Verification items for the finished model (mm, model axes). Face numbers are marked on the shaded views. A direction names the side the tool comes from. Give positions to 0.01 mm unless a question says otherwise; leave off trailing zeros. Order: outer loops, then holes, each group sorted by start corner. A loop starts at its lowest first (then second) coordinate and runs counter-clockwise, first axis right, second up. Notation, with made-up numbers: (-10.5, 23.5) -> (-1.5, 23.5) arc R5 ccw to (-1.5, 29.5) -> close; hole circle Ø11 at (89, 7.25). An arc over 180 degrees is marked (long way). Write each question's results on one line, items separated by ' | '. Start each with the question number.
1. Depth check by flat-ended pin: pin 1 Ø3 at (x, z) = (9.5, 8) entering from +Y; pin 2 Ø3 at (x, z) = (10.5, 1.5) entering from +Y; pin 3 Ø4 at (y, z) = (9, 2) entering from -X; pin 4 Ø2 at (x, z) = (10, 7) entering from +Y. Enter the tip coordinate at first touch or a pass-through.
2. Mould release check, pull along Y, two halves, no side actions. Record for the marked faces 4, 5, 6 and 7: +Y half, -Y half, draft (parallel to the pull), parting line (faces both ways), or undercut.
3. Cross-section at D-D, the plane y = 13. Enter the section's corners in (x, z).
4. Material ranges on L1, parallel to X at y = -13.05, z = 3; L2, parallel to X at y = -13.85, z = 3; L3, parallel to Z at x = -10, y = -13, recorded low to high. Write a range as from..to.
5. Cross-section at A-A, the plane x = 15. Enter the section's corners in (y, z).
6. Cross-section at C-C, the plane x = -10. Enter the section's corners in (y, z), then the cut area to 3 significant figures.
7. Cross-section at B-B, the plane z = 3. State how many separate pieces and enclosed holes the cut face has, then the cut area to 3 significant figures.
8. Set-up check for the marked faces 1, 2 and 3: record each of +Z, -Z, +X, -X, +Y, -Y from which the full face is reachable in a straight line by a thin tool's end or side.
from build123d import *

# Parameters (mm, degrees)
SKETCH1_R           = 4.5
BOSS_EXTRUDE1_DEPTH = 5
SKETCH2_W           = 5
SKETCH2_H           = 2.5
BOSS_EXTRUDE2_DEPTH = 5
SKETCH3_W           = 7.5
SKETCH3_H           = 2.5
BOSS_EXTRUDE3_DEPTH = 5
SKETCH4_W           = 7.5
SKETCH4_H           = 2.5
BOSS_EXTRUDE4_DEPTH = 5
SKETCH5_R           = 1.65
CUT_EXTRUDE1_DEPTH  = 5
FILLET1_R           = 2
FILLET2_R           = 2
FILLET3_R           = 2
FILLET4_R           = 10
FILLET5_R           = 5
FILLET6_R           = 1


with BuildPart() as part:
    # Sketch1 → Boss-Extrude1 (new body)
    with BuildSketch(Plane.XY):
        with BuildLine():
            Line((-7.5, 15), (-5.646592756, 12.528790341))
            ThreePointArc((-5.646592756, 12.528790341), (0, 16.5), (5.646592756, 12.528790341))
            Line((5.646592756, 12.528790341), (7.5, 15))
            Line((7.5, 15), (12.5, 15))
            Line((12.5, 15), (12.5, 10))
            Line((12.5, 10), (5, 0))
            Line((5, 0), (12.5, -10))
            Line((12.5, -10), (12.5, -15))
            Line((12.5, -15), (7.5, -15))
            Line((7.5, -15), (0, -5))
            Line((0, -5), (-7.5, -15))
            Line((-7.5, -15), (-12.5, -15))
            Line((-12.5, -15), (-12.5, -10))
            Line((-12.5, -10), (-5, 0))
            Line((-5, 0), (-12.5, 10))
            Line((-12.5, 10), (-12.5, 15))
            Line((-12.5, 15), (-7.5, 15))
        make_face()
        with Locations((0, 10.5)):
            Circle(SKETCH1_R, mode=Mode.SUBTRACT)
    extrude(amount=BOSS_EXTRUDE1_DEPTH)

    # Sketch2 → Boss-Extrude2 (add)
    with BuildSketch(Plane.XY.offset(5)):
        with Locations((-10, -13.75)):
            Rectangle(SKETCH2_W, SKETCH2_H)
        with Locations((10, -13.75)):
            Rectangle(SKETCH2_W, SKETCH2_H)
    extrude(amount=BOSS_EXTRUDE2_DEPTH)

    # Sketch3 → Boss-Extrude3 (add)
    with BuildSketch(Plane(origin=(12.5, 0, 0), x_dir=(0, 0, -1), z_dir=(1, 0, 0))):
        with Locations((-3.75, -13.75)):
            Rectangle(SKETCH3_W, SKETCH3_H)
    extrude(amount=BOSS_EXTRUDE3_DEPTH)

    # Sketch4 → Boss-Extrude4 (add)
    with BuildSketch(Plane.ZY.offset(12.5)):
        with Locations((3.75, -13.75)):
            Rectangle(SKETCH4_W, SKETCH4_H)
    extrude(amount=BOSS_EXTRUDE4_DEPTH)

    # Sketch5 → Cut-Extrude1 (cut)
    with BuildSketch(Plane(origin=(0, -12.5, 0), x_dir=(1, 0, 0), z_dir=(0, 1, 0))):
        with Locations((-15, -3)):
            Circle(SKETCH5_R)
        with Locations((15, -3)):
            Circle(SKETCH5_R)
        with Locations((-10, -7)):
            Circle(SKETCH5_R)
        with Locations((10, -7)):
            Circle(SKETCH5_R)
    extrude(amount=-CUT_EXTRUDE1_DEPTH, mode=Mode.SUBTRACT)

    # Fillet1
    fillet1_edges = [part.edges().sort_by_distance(p)[0] for p in [
        (12.5, -13.75, 7.5),
        (17.5, -13.75, 7.5),
        (-12.5, -13.75, 7.5),
        (-17.5, -13.75, 7.5),
    ]]
    fillet(fillet1_edges, radius=FILLET1_R)

    # Fillet2
    fillet2_edges = [part.edges().sort_by_distance(p)[0] for p in [
        (12.5, -13.75, 10),
        (7.5, -13.75, 10),
        (-7.5, -13.75, 10),
        (-12.5, -13.75, 10),
    ]]
    fillet(fillet2_edges, radius=FILLET2_R)

    # Fillet3
    fillet3_edges = [part.edges().sort_by_distance(p)[0] for p in [
        (-5.646592756, 12.528790341, 2.5),
        (5.646592756, 12.528790341, 2.5),
    ]]
    fillet(fillet3_edges, radius=FILLET3_R)

    # Fillet4
    fillet4_edges = [part.edges().sort_by_distance(p)[0] for p in [
        (5, 0, 2.5),
        (-5, 0, 2.5),
    ]]
    fillet(fillet4_edges, radius=FILLET4_R)

    # Fillet5
    fillet5_edges = [part.edges().sort_by_distance(p)[0] for p in [
        (0, -5, 2.5),
    ]]
    fillet(fillet5_edges, radius=FILLET5_R)

    # Fillet6
    fillet6_edges = [part.edges().sort_by_distance(p)[0] for p in [
        (-12.5, 10, 2.5),
        (-12.5, 15, 2.5),
        (-7.5, 15, 2.5),
        (12.5, 10, 2.5),
        (7.5, 15, 2.5),
        (12.5, 15, 2.5),
    ]]
    fillet(fillet6_edges, radius=FILLET6_R)


solid = part.part
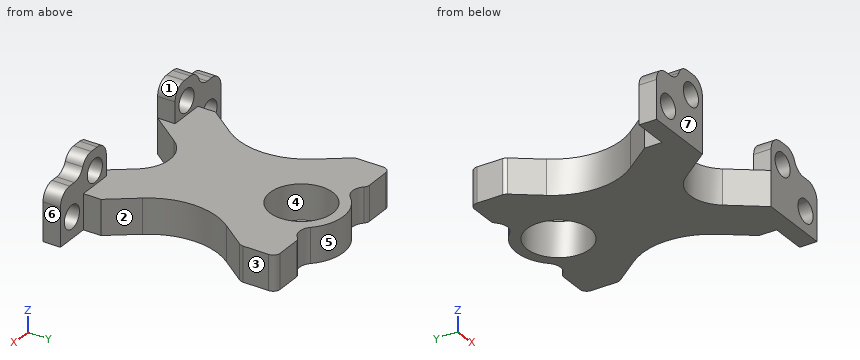
Results below:
1) pin 1: stops at y = -12.5 | pin 2: stops at y = 15 | pin 3: stops at x = -12.5 | pin 4: passes through
2) face 4: undercut | face 5: +Y half | face 6: draft | face 7: -Y half
3) outline: (-12.5, 0) -> (-3.74, 0) -> (-3.74, 5) -> (-12.5, 5) -> close; (3.74, 0) -> (12.5, 0) -> (12.5, 5) -> (3.74, 5) -> close
4) L1: x = -17.5..-16.65, -13.35..-6.04, 6.04..13.35, 16.65..17.5 | L2: x = -17.5..-16.65, -13.35..-6.64, 6.64..13.35, 16.65..17.5 | L3: z = 0..5.35, 8.65..10
5) outline: (-15, 0) -> (-12.5, 0) -> (-12.5, 1.35) -> (-15, 1.35) -> close; (-15, 4.65) -> (-12.5, 4.65) -> (-12.5, 7.5) -> (-15, 7.5) -> close
6) outline: (-15, 0) -> (-6.67, 0) -> (-6.67, 5) -> (-12.5, 5) -> (-12.5, 5.35) -> (-15, 5.35) -> close; (-15, 8.65) -> (-12.5, 8.65) -> (-12.5, 10) -> (-15, 10) -> close; (6.67, 0) -> (15, 0) -> (15, 5) -> (6.67, 5) -> close | area: 87.6 mm²
7) separate pieces: 3 | enclosed holes: 1 | area: 504 mm²
8) face 1: +Z, +Y, -Y | face 2: +Z, -Z, +X | face 3: +Z, -Z, +X, +Y
